The model under review builds one solid part; all positions refer to its coordinate system, in mm. Round coordinates to 2 decimals unless told otherwise and drop trailing zeros. Loops run counter-clockwise (first coordinate to the right, second up) from the corner with the lowest first, then second, coordinate; pieces in that order, holes last. Notation, with made-up numbers: (1, 79) -> (57, 79) arc R16 cw to (57, 102) -> close; hole circle Ø8 at (41, 8.25). An arc over 180 degrees is marked (long way). Write each question's results on one line, items separated by ' | '. Start each with the question number.
Item 1: We need section B-B (z = 2.8). Give the number of separate pieces and of enclosed holes in the cut face, and give its area (3 significant figures).
Item 2: Clearance check with flat-ended pins moving along their axes: pin 1 Ø2.5 at (y, z) = (-142, 1.5) entering from +X; pin 2 Ø7 at (x, y) = (120.65, -76.2) entering from +Z; pin 3 Ø1.5 at (x, z) = (-51.5, 2.5) entering from -Y; pin 4 Ø1.4 at (y, z) = (141.5, 3) entering from -X. State where each tip first meets the part, or that it passes through.
Item 3: For L1, parallel to Y at x = -207.3, z = 2.15; L2, parallel to Y at x = 120.65, z = 2.6; L3, parallel to X at y = -75.5, z = 4.35, list the stretches that pass through material, from the lowest coordinate up. Write a range as from..to.
Item 4: We need section A-A (x = -97). Give the boundary of the cut face in (y, z).
from build123d import *

# Parameters (mm, degrees)
SKETCH_1_W          = 500.8
SKETCH_1_H          = 300.8
EXTRUDE_1_DEPTH     = 4.75
SKETCH_2_R          = 3
SKETCH_2_W          = 25.4
SKETCH_2_H          = 25.4
CUT_EXTRUDE_1_DEPTH = 10
SKETCH_3_R          = 2.15
CUT_EXTRUDE_2_DEPTH = 5
SKETCH_4_R          = 2.15
CUT_EXTRUDE_3_DEPTH = 5
SKETCH_5_R          = 2.15
SKETCH_5_R_2        = 2.150000001
CUT_EXTRUDE_4_DEPTH = 5
SKETCH_7_R          = 2.15
SKETCH_7_R_2        = 2.150000004
CUT_EXTRUDE_6_DEPTH = 5
SKETCH_8_W          = 300
SKETCH_8_H          = 30
CUT_EXTRUDE_7_DEPTH = 10
FILLET_2_R          = 7


with BuildPart() as part:
    # 草圖1 → 填料-伸長1 (new body)
    with BuildSketch(Plane.XY):
        Rectangle(SKETCH_1_W, SKETCH_1_H)
    extrude(amount=EXTRUDE_1_DEPTH)

    # 草圖2 → 除料-伸長1 (cut)
    with BuildSketch(Plane(origin=(0, 0, 0), x_dir=(-1, 0, 0), z_dir=(0, 0, -1))):
        with Locations((-120.65, 76.2)):
            Circle(SKETCH_2_R)
        with Locations((-120.65, -76.2)):
            Circle(SKETCH_2_R)
        with Locations((120.65, -76.2)):
            Circle(SKETCH_2_R)
        with Locations((120.65, 76.2)):
            Circle(SKETCH_2_R)
        with Locations((-237.7, 137.7)):
            Rectangle(SKETCH_2_W, SKETCH_2_H)
        with Locations((-237.7, -137.7)):
            Rectangle(SKETCH_2_W, SKETCH_2_H)
        with Locations((237.7, 137.7)):
            Rectangle(SKETCH_2_W, SKETCH_2_H)
        with Locations((237.7, -137.7)):
            Rectangle(SKETCH_2_W, SKETCH_2_H)
    extrude(amount=-CUT_EXTRUDE_1_DEPTH, mode=Mode.SUBTRACT)

    # 草圖3 → 除料-伸長2 (cut)
    with BuildSketch(Plane.XY.offset(4.75)):
        with Locations((207.3, 137.7)):
            Circle(SKETCH_3_R)
        with Locations((182.8, 137.7)):
            Circle(SKETCH_3_R)
    extrude(amount=-CUT_EXTRUDE_2_DEPTH, mode=Mode.SUBTRACT)

    # 草圖4 → 除料-伸長3 (cut)
    with BuildSketch(Plane.XY.offset(4.75)):
        with Locations((237.7, 82.8)):
            Circle(SKETCH_4_R)
        with Locations((237.7, 107.3)):
            Circle(SKETCH_4_R)
    extrude(amount=-CUT_EXTRUDE_3_DEPTH, mode=Mode.SUBTRACT)

    # 草圖5 → 除料-伸長4 (cut)
    with BuildSketch(Plane.XY.offset(4.75)):
        with Locations((237.7, -107.300000014)):
            Circle(SKETCH_5_R)
        with Locations((237.7, -82.800000014)):
            Circle(SKETCH_5_R)
        with Locations((207.3, -137.7)):
            Circle(SKETCH_5_R_2)
        with Locations((182.8, -137.7)):
            Circle(SKETCH_5_R)
    extrude(amount=-CUT_EXTRUDE_4_DEPTH, mode=Mode.SUBTRACT)

    # 草圖7 → 除料-伸長6 (cut)
    with BuildSketch(Plane.XY.offset(4.75)):
        with Locations((-182.8, -137.7)):
            Circle(SKETCH_7_R)
        with Locations((-207.3, -137.7)):
            Circle(SKETCH_7_R)
        with Locations((-237.7, -107.3)):
            Circle(SKETCH_7_R)
        with Locations((-237.7, -82.8)):
            Circle(SKETCH_7_R)
        with Locations((-237.7, 82.800000014)):
            Circle(SKETCH_7_R_2)
        with Locations((-237.7, 107.300000014)):
            Circle(SKETCH_7_R_2)
        with Locations((-207.3, 137.7)):
            Circle(SKETCH_7_R)
        with Locations((-182.8, 137.7)):
            Circle(SKETCH_7_R)
    extrude(amount=-CUT_EXTRUDE_6_DEPTH, mode=Mode.SUBTRACT)

    # 草圖8 → 除料-伸長7 (cut)
    with BuildSketch(Plane(origin=(0, 0, 0), x_dir=(-1, 0, 0), z_dir=(0, 0, -1))):
        with Locations((0, -135.4)):
            Rectangle(SKETCH_8_W, SKETCH_8_H)
    extrude(amount=-CUT_EXTRUDE_7_DEPTH, mode=Mode.SUBTRACT)

    # 圓角2
    fillet_2_edges = [part.edges().sort_by_distance(p)[0] for p in [
        (150, -120.4, 2.375),
        (-150, -120.4, 2.375),
    ]]
    fillet(fillet_2_edges, radius=FILLET_2_R)


solid = part.part
Here are the results:
1) separate pieces: 1 | enclosed holes: 20 | area: 139,000 mm2
2) pin 1: stops at x = 225 | pin 2: stops at z = 4.75 | pin 3: stops at y = -120.4 | pin 4: stops at x = -225
3) L1: y = -150.4..-139.85, -135.55..135.55, 139.85..150.4 | L2: y = -120.4..-79.2, -73.2..73.2, 79.2..150.4 | L3: x = -250.4..-123.57, -117.73..117.73, 123.57..250.4
4) outline: (-120.4, 0) -> (150.4, 0) -> (150.4, 4.75) -> (-120.4, 4.75) -> close
